```python
from build123d import *

# Parameters (mm, degrees)
F0_W   = 18.0498287082
F0_H   = 60.3165104985
F0_W_2 = 13.8382017612
F0_W_3 = 17.7489968482
F0_H_2 = 11.1307352781
F2_R   = 2.5
F3_R   = 2.5
F4_R   = 2.5
F5_R   = 2.5


with BuildPart() as f1:
    # F0 (on Right) → F1 (revolve)
    with BuildSketch(Plane.YZ):
        with Locations((-44.2220792174, 30.1582552493)):
            Rectangle(F0_W, F0_H)
        with Locations((-28.2780639827, 30.1582552493)):
            Rectangle(F0_W_2, F0_H)
        with Locations((-12.484464678, 30.1582552493)):
            Rectangle(F0_W_3, F0_H)
        with Locations((-12.484464678, 65.8818781376)):
            Rectangle(F0_W_3, F0_H_2)
        with Locations((-44.2220792174, 65.8818781376)):
            Rectangle(F0_W, F0_H_2)
    revolve(axis=Axis((0, -28.4284799127, 0), (0, 1, 0)))

    # F2
    f2_edges = [f1.edges().sort_by_distance(p)[0] for p in [
        (0, -35.197165, -71.447246),
    ]]
    fillet(f2_edges, radius=F2_R)

    # F3
    f3_edges = [f1.edges().sort_by_distance(p)[0] for p in [
        (0, -21.358963, -71.447246),
    ]]
    fillet(f3_edges, radius=F3_R)

    # F4
    f4_edges = [f1.edges().sort_by_distance(p)[0] for p in [
        (0, -53.246994, -71.447246),
    ]]
    fillet(f4_edges, radius=F4_R)

    # F5
    f5_edges = [f1.edges().sort_by_distance(p)[0] for p in [
        (0, -3.609966, -71.447246),
    ]]
    fillet(f5_edges, radius=F5_R)


solid = f1.part
```
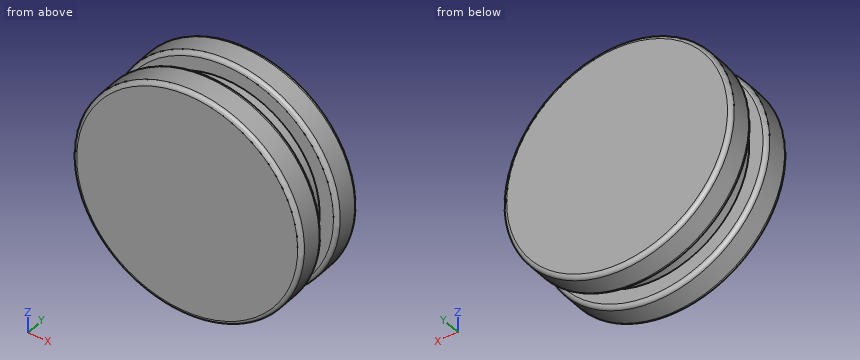
Could you check a few things on this model? Use its own coordinates, in mm. Round coordinates to 2 decimals unless told otherwise and drop trailing zeros. Loops run counter-clockwise (first coordinate to the right, second up) from the corner with the lowest first, then second, coordinate; pieces in that order, holes last. Notation, with made-up numbers: (-7.75, 63.5) - (27.25, 63.5) arc R23 cw to (27.25, 74.5) - close; hole circle Ø8 at (47, -39.75). An arc over 180 degrees is marked (long way). Answer in a Markdown table with one row per item. Add a question column.
(1) If we section it at C-C (y = -48.5): Please give me the cut outline in (x, z).
(2) If we section it at A-A (z = 0): Please give me the cut outline in (x, y).
(3) I'm going to push flat-ended pins straight in: pin 1 (12 mm diameter, centred on x = 13.5, y = -19, fed in from +Z); pin 2 (6 mm diameter, centred on x = -40, y = -19.5, fed in from +Z); pin 3 (2 mm diameter, centred on x = 48.5, y = -44, fed in from +Z). Where does each tip first touch, or does it pass through?
(4) I need wall thicknesses on line 1 along Y through (x, z) = (59, -25); line 2 along X through (y, z) = (-47, 4.5); line 3 along X through (y, z) = (-24.5, -39.5). Which ranges of each line are inside material? Lowest first, please.
(5) If we section it at B-B (x = 0): Please give me the cut outline in (y, z), plus the area to 3 significant figures.
(6) If we section it at D-D (y = -25): Please give me the cut outline in (x, z).
Model answer:
| question | item | result |
|---|---|---|
| 1 | outline | circle Ø142.89 at (0, 0) |
| 2 | outline | (-71.45, -50.75) arc R2.5 ccw to (-68.95, -53.25) - (68.95, -53.25) arc R2.5 ccw to (71.45, -50.75) - (71.45, -37.7) arc R2.5 ccw to (68.95, -35.2) - (60.32, -35.2) - (60.32, -21.36) - (68.95, -21.36) arc R2.5 ccw to (71.45, -18.86) - (71.45, -6.11) arc R2.5 ccw to (68.95, -3.61) - (-68.95, -3.61) arc R2.5 ccw to (-71.45, -6.11) - (-71.45, -18.86) arc R2.5 ccw to (-68.95, -21.36) - (-60.32, -21.36) - (-60.32, -35.2) - (-68.95, -35.2) arc R2.5 ccw to (-71.45, -37.7) - close |
| 3 | pin 1 | stops at z = 71.05 |
| 3 | pin 2 | stops at z = 61.09 |
| 3 | pin 3 | stops at z = 53.37 |
| 4 | line 1 | y = -53.25 to -35.2, -21.36 to -3.61 |
| 4 | line 2 | x = -71.31 to 71.31 |
| 4 | line 3 | x = -45.58 to 45.58 |
| 5 | outline | (-53.25, -68.95) arc R2.5 ccw to (-50.75, -71.45) - (-37.7, -71.45) arc R2.5 ccw to (-35.2, -68.95) - (-35.2, -60.32) - (-21.36, -60.32) - (-21.36, -68.95) arc R2.5 ccw to (-18.86, -71.45) - (-6.11, -71.45) arc R2.5 ccw to (-3.61, -68.95) - (-3.61, 68.95) arc R2.5 ccw to (-6.11, 71.45) - (-18.86, 71.45) arc R2.5 ccw to (-21.36, 68.95) - (-21.36, 60.32) - (-35.2, 60.32) - (-35.2, 68.95) arc R2.5 ccw to (-37.7, 71.45) - (-50.75, 71.45) arc R2.5 ccw to (-53.25, 68.95) - close |
| 5 | area | 6,770 mm² |
| 6 | outline | circle Ø120.63 at (0, 0) |
